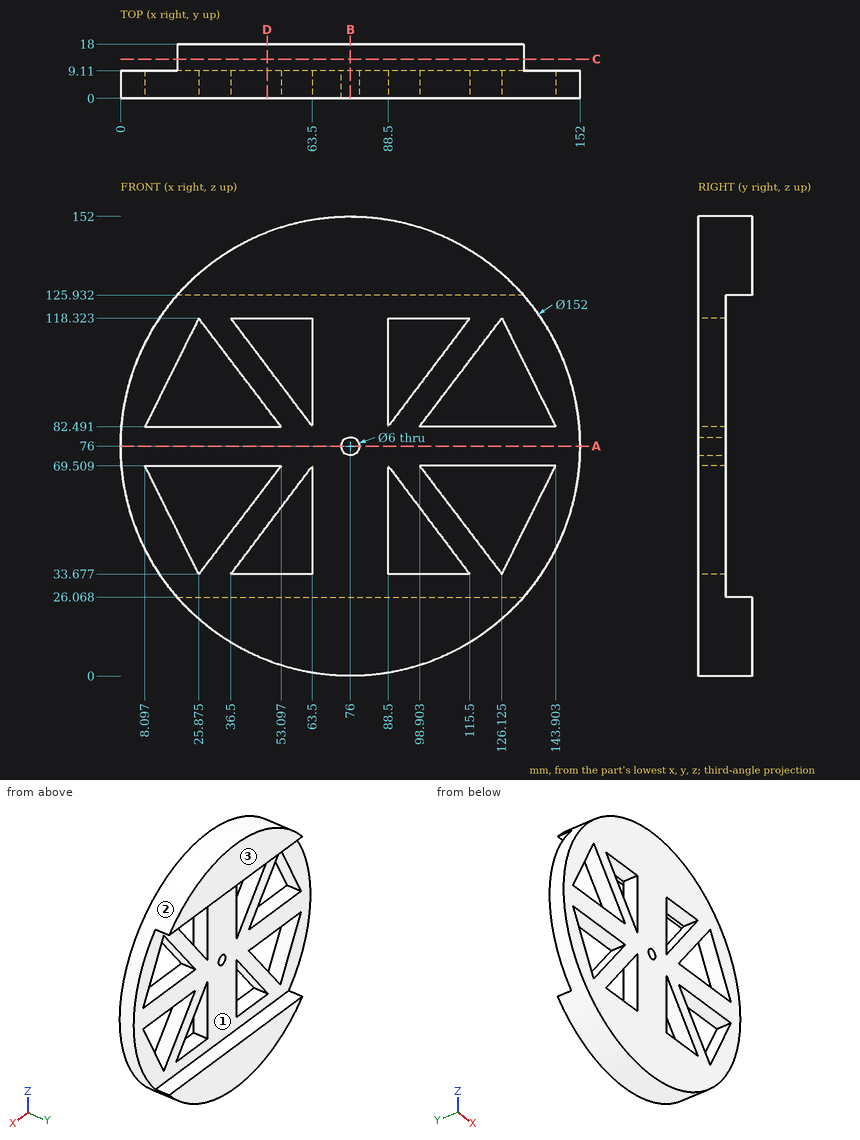
For this review, use the dimensioned drawing (mm, ordinates from the lowest corner) and the shaded views. Give positions to 0.01 mm unless a question says otherwise; leave off trailing zeros. Write each loop counter-clockwise with the first axis right and the second up, starting at its lowest first coordinate (ties: lowest second). Pieces come first, ordered by that corner, then holes. Notation, with made-up numbers: M -21.75,19.5 L 35.25,19.5 A22 cw 35.25,53.5 Z; hole C 59.25,-7 d1. An arc over 180 degrees is marked long. Answer as a JSON object with one key per item and string values. Group by question number.
Item 1: Draft analysis for pull direction Z (two halves, no side actions). For the marked faces 1, 2 and 3, state which applies: +Z half, -Z half, draft (parallel to the pull), parting line (faces both ways), or undercut.
Item 2: For pin 1 Ø7.5 at (x, y) = (48.5, 3.5) entering from -Z; pin 2 Ø2.5 at (x, y) = (89.5, 13) entering from -Z; pin 3 Ø4.5 at (x, y) = (128, 4) entering from +Z (1 decimal), all flat-tipped, find the tip position at first contact; note any pin that passes through.
Item 3: Consider section D-D on x = 48.5. Write out the cut boundary in (y, z).
Item 4: Consider section A-A on z = 76. Write out the cut boundary in (x, y), plus the area to 3 significant figures.
Item 5: Consider section C-C on y = 13. Write out the cut boundary in (x, z), plus the area to 3 significant figures.
Item 6: Consider section B-B on x = 76. Write out the cut boundary in (y, z), plus the area to 3 significant figures.
Item 7: For probe 1 along X at (y, z) = (2, 76); probe 2 along Z at (x, y) = (116.5, 8) (1 decimal); probe 3 along Z at (x, y) = (133, 2) (1 decimal), list the stretches that pass through material, from the lowest coordinate up. Write a range as [from, to].
Check result:
{
 "1": {"face 1": "undercut", "face 2": "parting line", "face 3": "draft"},
 "2": {"pin 1": "stops at z = 3.81", "pin 2": "stops at z = 0.99", "pin 3": "stops at z = 133.5"},
 "3": {"outline": "M 0,5.15 L 18,5.15 L 18,26.07 L 9.11,26.07 L 9.11,33.68 L 0,33.68 Z; M 0,49.6 L 9.11,49.6 L 9.11,63.46 L 0,63.46 Z; M 0,69.51 L 9.11,69.51 L 9.11,82.49 L 0,82.49 Z; M 0,88.54 L 9.11,88.54 L 9.11,102.4 L 0,102.4 Z; M 0,118.32 L 9.11,118.32 L 9.11,125.93 L 18,125.93 L 18,146.85 L 0,146.85 Z"},
 "4": {"outline": "M 0,0 L 73,0 L 73,9.11 L 0,9.11 Z; M 79,0 L 152,0 L 152,9.11 L 79,9.11 Z", "area": "1,330 mm^2"},
 "5": {"outline": "M 18.7,26.07 A76 ccw 133.3,26.07 Z; M 18.7,125.93 L 133.3,125.93 A76 ccw Z", "area": "4,140 mm^2"},
 "6": {"outline": "M 0,0 L 18,0 L 18,26.07 L 9.11,26.07 L 9.11,73 L 0,73 Z; M 0,79 L 9.11,79 L 9.11,125.93 L 18,125.93 L 18,152 L 0,152 Z", "area": "1,790 mm^2"},
 "7": {"probe 1": "x = [0, 73], [79, 152]", "probe 2": "z = [11.7, 46.3], [69.5, 82.5], [105.7, 140.3]", "probe 3": "z = [25.7, 47.5], [69.5, 82.5], [104.5, 126.3]"}
}
